```python
from build123d import *

# Parameters (mm, degrees)
CROQUIS1_W              = 30
CROQUIS1_H              = 20
SALIENTE_EXTRUIR1_DEPTH = 2
CROQUIS2_W              = 22
CROQUIS2_H              = 11
CROQUIS2_W_2            = 16
CROQUIS2_H_2            = 5
SALIENTE_EXTRUIR2_DEPTH = 120
CROQUIS3_W              = 16
CROQUIS3_H              = 5
CORTAR_EXTRUIR1_DEPTH   = 123


with BuildPart() as part:
    # Croquis1 → Saliente-Extruir1 (new body)
    with BuildSketch(Plane(origin=(0, 0, 0), x_dir=(1, 0, 0), z_dir=(0, 1, 0))):
        Rectangle(CROQUIS1_W, CROQUIS1_H)
    extrude(amount=SALIENTE_EXTRUIR1_DEPTH)

    # Croquis2 → Saliente-Extruir2 (add)
    with BuildSketch(Plane(origin=(0, 2, 0), x_dir=(1, 0, 0), z_dir=(0, 1, 0))):
        Rectangle(CROQUIS2_W, CROQUIS2_H)
        Rectangle(CROQUIS2_W_2, CROQUIS2_H_2, mode=Mode.SUBTRACT)
    extrude(amount=SALIENTE_EXTRUIR2_DEPTH)

    # Croquis3 → Cortar-Extruir1 (cut, through all)
    with BuildSketch(Plane(origin=(0, 122, 0), x_dir=(1, 0, 0), z_dir=(0, 1, 0))):
        Rectangle(CROQUIS3_W, CROQUIS3_H)
    extrude(amount=-CORTAR_EXTRUIR1_DEPTH, mode=Mode.SUBTRACT)


solid = part.part
```
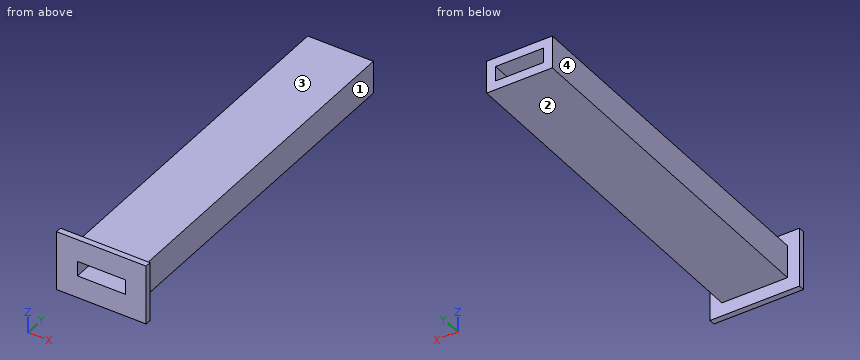
Could you check a few things on this model? Use its own coordinates, in mm. Face numbers are marked on the shaded views. A direction names the side the tool comes from. Round coordinates to 2 decimals unless told otherwise and drop trailing zeros. Write each loop counter-clockwise with the first axis right and the second up, starting at its lowest first coordinate (ties: lowest second). Pieces come first, ordered by that corner, then holes. Notation, with made-up numbers: M 25.5,84.5 L 57.5,84.5 A16 ccw 57.5,104.5 Z; hole C 4.5,80 d8. An arc over 180 degrees is marked long. Write each question's results on one line, items separated by ' | '. Start each with the question number.
1. Imagine slicing it at A-A on x = 6.25. List the corners of the cut face in (y, z) for me, and give its area (3 significant figures).
2. On a 3-axis mill with a long thin cutter (end or side, diameter ignored), from which of +Z, -Z, +X, -X, +Y, -Y can I reach the whole of each face in a straight line? I mean the marked faces 1, 2, 3 and 4. Say none if no direction works.
3. I need wall thicknesses on L1, parallel to Z at x = 5, y = 94; L2, parallel to X at y = 38.5, z = 1.25; L3, parallel to X at y = 43, z = -5. Which ranges of each line are inside material? Lowest first, please. Write a range as from..to.
4. Imagine slicing it at C-C on y = 114. List the corners of the cut face in (x, z) for me.
5. Imagine slicing it at B-B on z = 0.25. List the corners of the cut face in (x, y) for me, and give its area (3 significant figures).
6. I'm going to push flat-ended pins straight in: pin 1 Ø6 at (y, z) = (46.5, -2) entering from +X; pin 2 Ø6.5 at (x, y) = (-1, 92) entering from -Z; pin 3 Ø8 at (y, z) = (52.5, 6) entering from -X. Where does each tip first touch, or does it pass through?
7. Imagine slicing it at D-D on x = -12.25. List the corners of the cut face in (y, z) for me, and give its area (3 significant figures).
Result sheet:
1) outline: M 0,-10 L 2,-10 L 2,-5.5 L 122,-5.5 L 122,-2.5 L 0,-2.5 Z; M 0,2.5 L 122,2.5 L 122,5.5 L 2,5.5 L 2,10 L 0,10 Z | area: 750 mm^2
2) face 1: +Z, -Z, +X, +Y | face 2: -Z, +X, -X, +Y | face 3: +Z, +X, -X, +Y | face 4: +Z, -Z, -X, +Y
3) L1: z = -5.5..-2.5, 2.5..5.5 | L2: x = -11..-8, 8..11 | L3: x = -11..11
4) outline: M -11,-5.5 L 11,-5.5 L 11,5.5 L -11,5.5 Z; hole M -8,-2.5 L 8,-2.5 L 8,2.5 L -8,2.5 Z
5) outline: M -15,0 L -8,0 L -8,122 L -11,122 L -11,2 L -15,2 Z; M 8,0 L 15,0 L 15,2 L 11,2 L 11,122 L 8,122 Z | area: 748 mm^2
6) pin 1: stops at x = 11 | pin 2: stops at z = -5.5 | pin 3: stops at x = -11
7) outline: M 0,-10 L 2,-10 L 2,10 L 0,10 Z | area: 40.0 mm^2
